Could you check a few things on this model? Use its own coordinates, in mm. A direction names the side the tool comes from. Coordinates: 2 decimals unless noted, no trailing zeros. Order: outer loops, then holes, each group sorted by start corner. A loop starts at its lowest first (then second) coordinate and runs counter-clockwise, first axis right, second up. Notation, with made-up numbers: (40.5, 24) -> (61.5, 24) arc R15 ccw to (61.5, 46) -> close; hole circle Ø7 at (45, -29). An arc over 180 degrees is marked (long way). Use a Markdown table: item, result. Add a question column.
1) Will these pins go through, and if not, where does the flat tip stop? pin 1 Ø13 at (x, y) = (7.5, 95.5) entering from +Z; pin 2 Ø2 at (x, y) = (53, 1) entering from +Z; pin 3 Ø4.5 at (y, z) = (110, 10.5) entering from -X; pin 4 Ø3.5 at (x, y) = (95.5, 94) entering from +Z.
2) If we section it at C-C (x = 40): Write out the boundary of the cut face in (y, z).
3) If we section it at A-A (x = 7): Write out the boundary of the cut face in (y, z).
4) Thinking about a two-plate mould opening in X: for faces 1 (the flat face through (53, 53, 0)), 2 (the flat face through (51, 53, 2)), 3 (the cylindrical face through (1.141, 1.203, 9.367)), 4 (the cylindrical face through (6.6, 95.4, 2.5)), which applies, +X half, -X half, draft (parallel to the pull), parting line (faces both ways), or undercut?
5) If we section it at B-B (z = 14): Give the number of separate pieces and of enclosed holes in the cut face, plus the area to 3 significant figures.
6) If I drill on L1, parallel to X at y = 97, z = 3.6; L2, parallel to Y at x = 97, z = 1.5; L3, parallel to Y at x = 87, z = 2.5, over which ranges is the centre line in solid material (lowest first)? Write a range as [from, to].
7) Which directions (+Z, -Z, +X, -X, +Y, -Y) give clear straight access to the entire face, cutting with the end or side of a thin tool? Please do faces 5 (the cylindrical face through (1.203, 102.859, 9.367)), 6 (the flat face through (51, 0, 5)), 7 (the flat face through (96, 95, 5)).
```python
from build123d import *

# Parameters (mm, degrees)
SKETCH_1_R          = 1.65
EXTRUDE_1_DEPTH     = 2
SKETCH_2_R          = 7
SKETCH_2_R_2        = 1.65
EXTRUDE_2_DEPTH     = 3
EXTRUDE_3_DEPTH     = 17
EXTRUDE_4_DEPTH     = 19
SKETCH_6_R          = 1.65
CUT_EXTRUDE_1_DEPTH = 10
SKETCH_7_W          = 77
SKETCH_7_H          = 2
CUT_EXTRUDE_2_DEPTH = 10
SKETCH_8_W          = 25
SKETCH_8_H          = 10
CUT_EXTRUDE_3_DEPTH = 10
SKETCH_9_R          = 1.4
CUT_EXTRUDE_4_DEPTH = 22
SKETCH_10_R         = 1.4
CUT_EXTRUDE_5_DEPTH = 22


with BuildPart() as part:
    # 草图1 → 凸台-拉伸1 (new body)
    with BuildSketch(Plane.XY):
        with BuildLine():
            Line((4, 0), (100, 0))
            ThreePointArc((100, 0), (102.828427125, 1.171572875), (104, 4))
            Line((104, 4), (104, 100))
            ThreePointArc((104, 100), (102.828427125, 102.828427125), (100, 104))
            Line((100, 104), (4, 104))
            ThreePointArc((4, 104), (1.171572875, 102.828427125), (0, 100))
            Line((0, 100), (0, 4))
            ThreePointArc((0, 4), (1.171572875, 1.171572875), (4, 0))
        make_face()
        with Locations((7, 97)):
            Circle(SKETCH_1_R, mode=Mode.SUBTRACT)
        with Locations((97, 97)):
            Circle(SKETCH_1_R, mode=Mode.SUBTRACT)
        with Locations((7, 7)):
            Circle(SKETCH_1_R, mode=Mode.SUBTRACT)
        with Locations((97, 7)):
            Circle(SKETCH_1_R, mode=Mode.SUBTRACT)
    extrude(amount=EXTRUDE_1_DEPTH)

    # 草图2 → 凸台-拉伸2 (add)
    # profile 1 of 4: a face of its own
    with BuildSketch(Plane.XY.offset(2)):
        with Locations(Location((7, 7, 0), (0, 0, 180))):
            Circle(SKETCH_2_R)
        with Locations((7, 7)):
            Circle(SKETCH_2_R_2, mode=Mode.SUBTRACT)
    # profile 2 of 4: a face of its own
    with BuildSketch(Plane.XY.offset(2)):
        with Locations((97, 7)):
            Circle(SKETCH_2_R)
        with Locations((97, 7)):
            Circle(SKETCH_2_R_2, mode=Mode.SUBTRACT)
    # profile 3 of 4: a face of its own
    with BuildSketch(Plane.XY.offset(2)):
        with Locations(Location((7, 97, 0), (0, 0, 180))):
            Circle(SKETCH_2_R)
        with Locations((7, 97)):
            Circle(SKETCH_2_R_2, mode=Mode.SUBTRACT)
    # profile 4 of 4: a face of its own
    with BuildSketch(Plane.XY.offset(2)):
        with Locations((97, 97)):
            Circle(SKETCH_2_R)
        with Locations((97, 97)):
            Circle(SKETCH_2_R_2, mode=Mode.SUBTRACT)
    extrude(amount=EXTRUDE_2_DEPTH)

    # 草图3 → 凸台-拉伸3 (add)
    with BuildSketch(Plane.XY.offset(2)):
        with BuildLine():
            Line((100, 104), (4, 104))
            ThreePointArc((4, 104), (1.171572875, 102.828427125), (0, 100))
            Line((0, 100), (0, 4))
            ThreePointArc((0, 4), (1.171572875, 1.171572875), (4, 0))
            Line((4, 0), (100, 0))
            ThreePointArc((100, 0), (102.828427125, 1.171572875), (104, 4))
            Line((104, 4), (104, 100))
            ThreePointArc((104, 100), (102.828427125, 102.828427125), (100, 104))
        make_face()
        with BuildLine():
            Line((100, 102), (4, 102))
            ThreePointArc((4, 102), (2.585786438, 101.414213562), (2, 100))
            Line((2, 100), (2, 4))
            ThreePointArc((2, 4), (2.585786438, 2.585786438), (4, 2))
            Line((4, 2), (100, 2))
            ThreePointArc((100, 2), (101.414213562, 2.585786438), (102, 4))
            Line((102, 4), (102, 100))
            ThreePointArc((102, 100), (101.414213562, 101.414213562), (100, 102))
        make_face(mode=Mode.SUBTRACT)
    extrude(amount=EXTRUDE_3_DEPTH)

    # 草图5 → 凸台-拉伸4 (add, through all)
    with BuildSketch(Plane.XY.offset(19)):
        with BuildLine():
            Line((104, 4), (104, -15))
            Line((104, -15), (100, -15))
            Line((100, -15), (100, 0))
            ThreePointArc((100, 0), (102.828427125, 1.171572875), (104, 4))
        make_face()
        with BuildLine():
            Line((104, 100), (104, 119))
            Line((104, 119), (100, 119))
            Line((100, 119), (100, 104))
            ThreePointArc((100, 104), (102.828427125, 102.828427125), (104, 100))
        make_face()
    extrude(amount=-EXTRUDE_4_DEPTH)

    # 草图6 → 切除-拉伸1 (cut)
    with BuildSketch(Plane.ZY.offset(-100)):
        with Locations(Location((10, -7.5, 0), (0, 0, 270))):
            Circle(SKETCH_6_R)
        with Locations(Location((10, 111.5, 0), (0, 0, 270))):
            Circle(SKETCH_6_R)
    extrude(amount=-CUT_EXTRUDE_1_DEPTH, mode=Mode.SUBTRACT)

    # 草图7 → 切除-拉伸2 (cut)
    with BuildSketch(Plane.XY.offset(19)):
        with Locations((53.5, 1)):
            Rectangle(SKETCH_7_W, SKETCH_7_H)
    extrude(amount=-CUT_EXTRUDE_2_DEPTH, mode=Mode.SUBTRACT)

    # 草图8 → 切除-拉伸3 (cut)
    with BuildSketch(Plane(origin=(0, 104, 0), x_dir=(1, 0, 0), z_dir=(0, 1, 0))):
        with Locations((67.5, -14)):
            Rectangle(SKETCH_8_W, SKETCH_8_H)
    extrude(amount=-CUT_EXTRUDE_3_DEPTH, mode=Mode.SUBTRACT)

    # 草图9 → 切除-拉伸4 (cut)
    with BuildSketch(Plane(origin=(0, 104, 0), x_dir=(1, 0, 0), z_dir=(0, 1, 0))):
        with Locations(Location((40, -14, 0), (0, 0, 270))):
            Circle(SKETCH_9_R)
    extrude(amount=-CUT_EXTRUDE_4_DEPTH, mode=Mode.SUBTRACT)

    # 草图10 → 切除-拉伸5 (cut)
    with BuildSketch(Plane.ZY):
        with Locations((14, 30)):
            Circle(SKETCH_10_R)
    extrude(amount=-CUT_EXTRUDE_5_DEPTH, mode=Mode.SUBTRACT)


solid = part.part
```
Answer sheet:
| question | item | result |
|---|---|---|
| 1 | pin 1 | z = 19 |
| 1 | pin 2 | z = 9 |
| 1 | pin 3 | x = 100 |
| 1 | pin 4 | z = 5 |
| 2 | outline | (0, 0) -> (104, 0) -> (104, 12.6) -> (102, 12.6) -> (102, 2) -> (2, 2) -> (2, 9) -> (0, 9) -> close; (102, 15.4) -> (104, 15.4) -> (104, 19) -> (102, 19) -> close |
| 3 | outline | (0, 0) -> (5.35, 0) -> (5.35, 5) -> (2, 5) -> (2, 19) -> (0, 19) -> close; (8.65, 0) -> (95.35, 0) -> (95.35, 5) -> (90, 5) -> (90, 2) -> (14, 2) -> (14, 5) -> (8.65, 5) -> close; (98.65, 0) -> (104, 0) -> (104, 19) -> (102, 19) -> (102, 5) -> (98.65, 5) -> close |
| 4 | face 1 | draft |
| 4 | face 2 | undercut |
| 4 | face 3 | -X half |
| 4 | face 4 | undercut |
| 5 | separate pieces | 4 |
| 5 | enclosed holes | 0 |
| 5 | area | 717 mm2 |
| 6 | L1 | [0, 5.35], [8.65, 14], [90, 95.35], [98.65, 104] |
| 6 | L2 | [0, 5.35], [8.65, 95.35], [98.65, 104] |
| 6 | L3 | [0, 2], [102, 104] |
| 7 | face 5 | +Z, -Z, -X, +Y |
| 7 | face 6 | +Z, -Z, -X, -Y |
| 7 | face 7 | +Z |
